Check sheet for the modelled part. Datum: model origin and axes. Units: mm. Face numbers are marked on the shaded views. Round coordinates to 2 decimals unless told otherwise and drop trailing zeros. Answer as a JSON object with one key per item and string values. Group by question number.
Item 1: Thickness scan on line 1 (X direction, y = 0, z = 1); line 2 (Y direction, x = 0, z = 1.5); line 3 (Y direction, x = 0, z = 1.65). Record the ranges inside material, lowest first.
Item 2: Gauge pin test, flat ends, axial feed: P1, Ø4, axis at x = -4.5, z = 2, coming from the -Y side; P2, Ø2.5, axis at x = 0, y = 0, coming from the -Z side; P3, Ø4, axis at x = 3, y = -1.5, coming from the +Z side; P4, Ø5, axis at x = -2, y = 6.5, coming from the -Z side. Record the tip position at first contact, or that the pin passes through.
Item 3: Release check for a two-part mould opening along Y. For the marked faces 1, 2 and 3 record: pulls with the +Y half, pulls with the -Y half, needs draft (parallel to the pull), parting line crosses it, or undercut.
```python
from build123d import *

# Parameters (mm, degrees)
F3_DEPTH = 25
F4_R     = 10
F5_R     = 2


with BuildPart() as f1:
    # F0 (on Front) → F1 (revolve)
    with BuildSketch(Plane.XZ):
        with BuildLine():
            Line((0, 5.5), (1.5, 4))
            Line((1.5, 4), (1.5, 0))
            Line((1.5, 0), (8, 0))
            ThreePointArc((8, 0), (5.6568542495, 5.6568542495), (0, 8))
            Line((0, 8), (0, 5.5))
        make_face()
    revolve(axis=Axis((0, 0, 2.75), (0, 0, -1)))

    # F2 (on Top) → F3 (cut)
    with BuildSketch(Plane.XY):
        Polygon((28.3564090981, 0), (0, -5), (-28.3564090981, 0), (-28.3564090981, -16.375022141), (0, -16.375022141), (28.3564090981, -16.375022141), align=None)
    extrude(amount=F3_DEPTH, mode=Mode.SUBTRACT)

    # F4
    f4_edges = [f1.edges().sort_by_distance(p)[0] for p in [
        (0, -5, 3.122499),
    ]]
    fillet(f4_edges, radius=F4_R)

    # F5
    f5_edges = [f1.edges().sort_by_distance(p)[0] for p in [
        (-5.546967, -4.02192, 4.129808),
    ]]
    fillet(f5_edges, radius=F5_R)


solid = f1.part
```
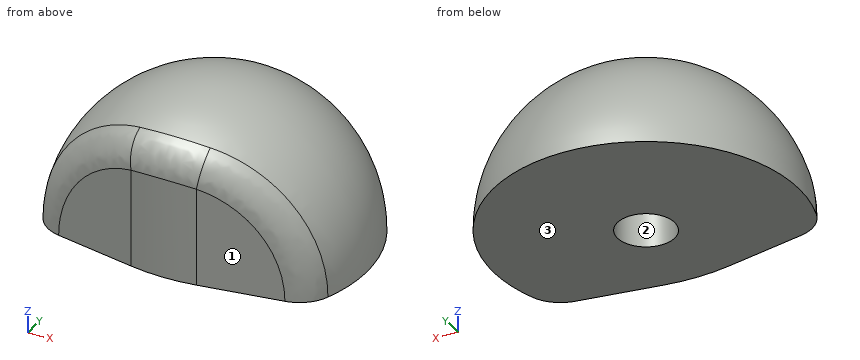
Completed:
{
 "1": {"line 1": "-7.94 to -1.5, 1.5 to 7.94", "line 2": "-4.85 to -1.5, 1.5 to 7.86", "line 3": "-4.85 to -1.5, 1.5 to 7.83"},
 "2": {"P1": "y = -4.56", "P2": "z = 4.25", "P3": "z = 7.88", "P4": "z = 0"},
 "3": {"face 1": "pulls with the -Y half", "face 2": "undercut", "face 3": "needs draft"}
}
